Could you check a few things on this model? Use its own coordinates, in mm. Face numbers are marked on the shaded views. Round coordinates to 2 decimals unless told otherwise and drop trailing zeros. Write each loop counter-clockwise with the first axis right and the second up, starting at its lowest first coordinate (ties: lowest second). Pieces come first, ordered by that corner, then holes. Notation, with made-up numbers: (43.5, 47) -> (81.5, 47) arc R20 ccw to (81.5, 58) -> close; hole circle Ø11 at (48, 23). An arc over 180 degrees is marked (long way). Answer as CSV lines item,"result". Start each with the question number.
Q1. If I drill on line 1 (Z direction, x = 0, y = -6.75); line 2 (X direction, y = -7.75, z = 16.25); line 3 (X direction, y = -7, z = 3.5), over which ranges is the centre line in solid material (lowest first)? Write a range as [from, to].
Q2. Will these pins go through, and if not, where does the flat tip stop? pin 1 Ø5 at (x, z) = (-12.5, 4.5) entering from +Y; pin 2 Ø5 at (x, z) = (13, 3) entering from -Y; pin 3 Ø1.8 at (x, z) = (0, 14) entering from -Y; pin 4 Ø2 at (y, z) = (6, 5) entering from +X.
Q3. Imagine slicing it at B-B on y = -6.75. Please give me the cut outline in (x, z).
Q4. Imagine slicing it at A-A on z = 14. Please give me the cut outline in (x, y).
Q5. If we mould it in two halves opening along Z, with no side actions, what happens to the marked faces 1, 2 and 3? For each: pulls with the +Z half, pulls with the -Z half, needs draft (parallel to the pull), parting line crosses it, or undercut.
Q6. Imagine slicing it at D-D on x = -12. Please give me the cut outline in (y, z).
Q7. Imagine slicing it at C-C on x = 0. Please give me the cut outline in (y, z), and give its area (3 significant figures).
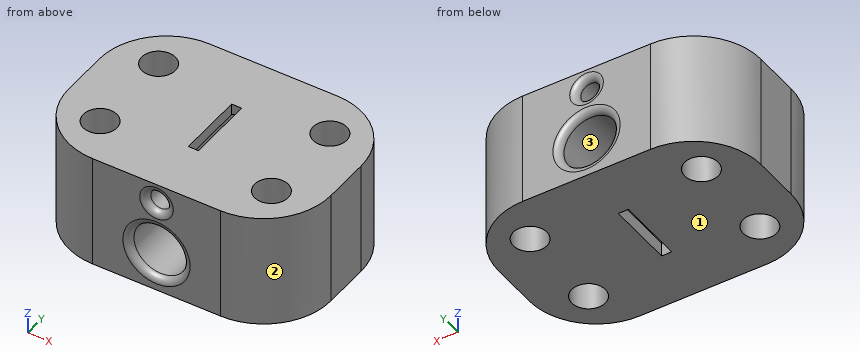
from build123d import *

# Parameters (mm, degrees)
F0_W      = 39
F0_H      = 27
F1_DEPTH  = 17
F2_R      = 10
F3_R      = 2.5
F4_DEPTH  = 17.001
F5_R      = 1.5
F6_DEPTH  = 27.001
F7_W      = 1.5
F7_H      = 10
F8_DEPTH  = 1.7019618943
F9_R      = 4
F10_DEPTH = 27.001
F11_R     = 1
F12_W     = 1.5
F12_H     = 10
F13_DEPTH = 2.0719415886


with BuildPart() as f1:
    # F0 (on Top) → F1 (new body)
    with BuildSketch(Plane.XY):
        Rectangle(F0_W, F0_H)
    extrude(amount=F1_DEPTH)

    # F2
    f2_edges = [f1.edges().sort_by_distance(p)[0] for p in [
        (19.5, 13.5, 8.5),
        (-19.5, 13.5, 8.5),
        (-19.5, -13.5, 8.5),
        (19.5, -13.5, 8.5),
    ]]
    fillet(f2_edges, radius=F2_R)

    # F3 (on face) → F4 (cut, through all)
    with BuildSketch(Plane.XY.offset(17)):
        with Locations((-12.75, -6.75)):
            Circle(F3_R)
        with Locations((12.75, 6.75)):
            Circle(F3_R)
        with Locations((12.75, -6.75)):
            Circle(F3_R)
        with Locations((-12.75, 6.75)):
            Circle(F3_R)
    extrude(amount=-F4_DEPTH, mode=Mode.SUBTRACT)

    # F5 (on face) → F6 (cut, through all)
    with BuildSketch(Plane.XZ.offset(13.5)):
        with Locations((0, 14)):
            Circle(F5_R)
    extrude(amount=-F6_DEPTH, mode=Mode.SUBTRACT)

    # F7 (on face) → F8 (cut, through all)
    with BuildSketch(Plane.XY.offset(17)):
        Rectangle(F7_W, F7_H)
    extrude(amount=-F8_DEPTH, mode=Mode.SUBTRACT)

    # F9 (on face) → F10 (cut, through all)
    with BuildSketch(Plane.XZ.offset(13.5)):
        with Locations((0, 6)):
            Circle(F9_R)
    extrude(amount=-F10_DEPTH, mode=Mode.SUBTRACT)

    # F11
    f11_edges = [f1.edges().sort_by_distance(p)[0] for p in [
        (-1.5, -13.5, 14),
        (-1.5, 13.5, 14),
        (-4, -13.5, 6),
        (-4, 13.5, 6),
    ]]
    fillet(f11_edges, radius=F11_R)

    # F12 (on face) → F13 (cut, through all)
    with BuildSketch(Plane(origin=(0, 0, 0), x_dir=(1, 0, 0), z_dir=(0, 0, -1))):
        Rectangle(F12_W, F12_H)
    extrude(amount=-F13_DEPTH, mode=Mode.SUBTRACT)


solid = f1.part
Checks:
1,line 1,"[0, 2], [10, 12.5], [15.5, 17]"
1,line 2,"[-18.55, -15.04], [-10.46, 10.46], [15.04, 18.55]"
1,line 3,"[-18.87, -15.24], [-10.26, -3.12], [3.12, 10.26], [15.24, 18.87]"
2,pin 1,"y = 13.49"
2,pin 2,"y = -13.45"
2,pin 3,"through"
2,pin 4,"x = 19.39"
3,outline,"(-18.96, 0) -> (-15.25, 0) -> (-15.25, 17) -> (-18.96, 17) -> close; (-10.25, 0) -> (10.25, 0) -> (10.25, 17) -> (-10.25, 17) -> close; (15.25, 0) -> (18.96, 0) -> (18.96, 17) -> (15.25, 17) -> close; hole circle Ø8 at (0, 6); hole circle Ø3 at (0, 14)"
4,outline,"(-19.5, -3.5) arc R10 ccw to (-9.5, -13.5) -> (-2.5, -13.5) arc R1 ccw to (-1.5, -12.5) -> (-1.5, 12.5) arc R1 ccw to (-2.5, 13.5) -> (-9.5, 13.5) arc R10 ccw to (-19.5, 3.5) -> close; (1.5, -12.5) arc R1 ccw to (2.5, -13.5) -> (9.5, -13.5) arc R10 ccw to (19.5, -3.5) -> (19.5, 3.5) arc R10 ccw to (9.5, 13.5) -> (2.5, 13.5) arc R1 ccw to (1.5, 12.5) -> close; hole circle Ø5 at (-12.75, -6.75); hole circle Ø5 at (-12.75, 6.75); hole circle Ø5 at (12.75, -6.75); hole circle Ø5 at (12.75, 6.75)"
5,face 1,"pulls with the -Z half"
5,face 2,"needs draft"
5,face 3,"undercut"
6,outline,"(-13.18, 0) -> (-9.13, 0) -> (-9.13, 17) -> (-13.18, 17) -> close; (-4.37, 0) -> (4.37, 0) -> (4.37, 17) -> (-4.37, 17) -> close; (9.13, 0) -> (13.18, 0) -> (13.18, 17) -> (9.13, 17) -> close"
7,outline,"(-13.5, 0) -> (-5, 0) -> (-5, 2) -> (-12.5, 2) arc R1 ccw to (-13.5, 1) -> close; (-13.5, 11) arc R1 ccw to (-12.5, 10) -> (12.5, 10) arc R1 ccw to (13.5, 11) -> (13.5, 11.5) arc R1 ccw to (12.5, 12.5) -> (-12.5, 12.5) arc R1 ccw to (-13.5, 11.5) -> close; (-13.5, 16.5) arc R1 ccw to (-12.5, 15.5) -> (-5, 15.5) -> (-5, 17) -> (-13.5, 17) -> close; (5, 0) -> (13.5, 0) -> (13.5, 1) arc R1 ccw to (12.5, 2) -> (5, 2) -> close; (5, 15.5) -> (12.5, 15.5) arc R1 ccw to (13.5, 16.5) -> (13.5, 17) -> (5, 17) -> close"
7,area,"125 mm^2"
